```python
from build123d import *

# Parameters (mm, degrees)
SKETCH1_W                = 31
SKETCH1_H                = 14
BOSS_EXTRUDE1_DEPTH      = 6.6
SKETCH2_R                = 2.3
CUT_EXTRUDE1_DEPTH       = 1
ZAOBLIT7_R               = 3.3
ZAOBLIT12_R              = 3.3
ZAOBLIT13_R              = 3.3
ZAOBLIT14_R              = 3.3
ODEBRAT_START            = -1
SKICA1_R                 = 2.3
ODEBRAT_VYSUNUT_M1_DEPTH = 1
SKICA3_R                 = 2.3
ODEBRAT_VYSUNUT_M2_DEPTH = 3
ODEBRAT_VYSUNUT_M2_DRAFT = -15
SKICA4_R                 = 2.3
ODEBRAT_VYSUNUT_M3_DEPTH = 3
ODEBRAT_VYSUNUT_M3_DRAFT = -15
SKICA5_R                 = 2.3
ODEBRAT_VYSUNUT_M4_DEPTH = 3
ODEBRAT_VYSUNUT_M4_DRAFT = -15
SKICA6_R                 = 2.3
ODEBRAT_VYSUNUT_M5_DEPTH = 3
ODEBRAT_VYSUNUT_M5_DRAFT = -15


with BuildPart() as part:
    # Sketch1 → Boss-Extrude1 (new body)
    with BuildSketch(Plane.XY):
        with Locations((15.5, 7)):
            Rectangle(SKETCH1_W, SKETCH1_H)
    extrude(amount=BOSS_EXTRUDE1_DEPTH)

    # Sketch2 → Cut-Extrude1 (cut)
    with BuildSketch(Plane.ZY):
        with Locations((3.3, 10.7)):
            Circle(SKETCH2_R)
        with Locations((3.3, 3.3)):
            Circle(SKETCH2_R)
    extrude(amount=-CUT_EXTRUDE1_DEPTH, mode=Mode.SUBTRACT)

    # Zaoblit7
    zaoblit7_edges = [part.edges().sort_by_distance(p)[0] for p in [
        (15.5, 14, 0),
    ]]
    fillet(zaoblit7_edges, radius=ZAOBLIT7_R)

    # Zaoblit12
    zaoblit12_edges = [part.edges().sort_by_distance(p)[0] for p in [
        (15.5, 14, 6.6),
    ]]
    fillet(zaoblit12_edges, radius=ZAOBLIT12_R - 0.0001)  # a hair under: the kernel refuses the full size

    # Zaoblit13
    zaoblit13_edges = [part.edges().sort_by_distance(p)[0] for p in [
        (15.5, 0, 6.6),
    ]]
    fillet(zaoblit13_edges, radius=ZAOBLIT13_R)

    # Zaoblit14
    zaoblit14_edges = [part.edges().sort_by_distance(p)[0] for p in [
        (15.5, 0, 0),
    ]]
    fillet(zaoblit14_edges, radius=ZAOBLIT14_R - 0.0001)  # a hair under: the kernel refuses the full size

    # Skica1 → Odebrat vysunutím1 (cut)
    with BuildSketch(Plane(origin=(31, 0, 0), x_dir=(0, 0, -1), z_dir=(1, 0, 0)).offset(ODEBRAT_START)):
        with Locations(Location((-3.3, 10.7, 0), (0, 0, 180))):
            Circle(SKICA1_R)
        with Locations(Location((-3.3, 3.3, 0), (0, 0, 180))):
            Circle(SKICA1_R)
    extrude(amount=ODEBRAT_VYSUNUT_M1_DEPTH, mode=Mode.SUBTRACT)


with BuildPart() as odebrat_vysunut_m2_tool:
    # Skica3 → Odebrat vysunutím2 (with draft: the straight prism first)
    with BuildSketch(Plane.ZY.offset(-1)):
        with Locations((3.3, 10.7)):
            Circle(SKICA3_R)
    extrude(amount=-ODEBRAT_VYSUNUT_M2_DEPTH)
    # Odebrat vysunutím2: the draft: its side faces are tilted about the plane it starts from
    odebrat_vysunut_m2_sides = [odebrat_vysunut_m2_tool.faces().sort_by_distance(p)[0] for p in [
        (2.5, 10.7, 1),
    ]]
    draft(odebrat_vysunut_m2_sides, Plane.ZY.offset(-1), ODEBRAT_VYSUNUT_M2_DRAFT)


with BuildPart() as part_1:
    add(part.part)

    # Odebrat vysunutím2: cut by odebrat_vysunut_m2_tool
    add(odebrat_vysunut_m2_tool.part, mode=Mode.SUBTRACT)


with BuildPart() as odebrat_vysunut_m3_tool:
    # Skica4 → Odebrat vysunutím3 (with draft: the straight prism first)
    with BuildSketch(Plane.ZY.offset(-1)):
        with Locations((3.3, 3.3)):
            Circle(SKICA4_R)
    extrude(amount=-ODEBRAT_VYSUNUT_M3_DEPTH)
    # Odebrat vysunutím3: the draft: its side faces are tilted about the plane it starts from
    odebrat_vysunut_m3_sides = [odebrat_vysunut_m3_tool.faces().sort_by_distance(p)[0] for p in [
        (2.5, 3.3, 1),
    ]]
    draft(odebrat_vysunut_m3_sides, Plane.ZY.offset(-1), ODEBRAT_VYSUNUT_M3_DRAFT)


with BuildPart() as part_2:
    add(part_1.part)

    # Odebrat vysunutím3: cut by odebrat_vysunut_m3_tool
    add(odebrat_vysunut_m3_tool.part, mode=Mode.SUBTRACT)


with BuildPart() as odebrat_vysunut_m4_tool:
    # Skica5 → Odebrat vysunutím4 (with draft: the straight prism first)
    with BuildSketch(Plane(origin=(30, 0, 0), x_dir=(0, 0, -1), z_dir=(1, 0, 0))):
        with Locations(Location((-3.3, 10.7, 0), (0, 0, 180))):
            Circle(SKICA5_R)
    extrude(amount=-ODEBRAT_VYSUNUT_M4_DEPTH)
    # Odebrat vysunutím4: the draft: its side faces are tilted about the plane it starts from
    odebrat_vysunut_m4_sides = [odebrat_vysunut_m4_tool.faces().sort_by_distance(p)[0] for p in [
        (28.5, 10.7, 1),
    ]]
    draft(odebrat_vysunut_m4_sides, Plane(origin=(30, 0, 0), x_dir=(0, 0, -1), z_dir=(1, 0, 0)), ODEBRAT_VYSUNUT_M4_DRAFT)


with BuildPart() as part_3:
    add(part_2.part)

    # Odebrat vysunutím4: cut by odebrat_vysunut_m4_tool
    add(odebrat_vysunut_m4_tool.part, mode=Mode.SUBTRACT)


with BuildPart() as odebrat_vysunut_m5_tool:
    # Skica6 → Odebrat vysunutím5 (with draft: the straight prism first)
    with BuildSketch(Plane(origin=(30, 0, 0), x_dir=(0, 0, -1), z_dir=(1, 0, 0))):
        with Locations(Location((-3.3, 3.3, 0), (0, 0, 180))):
            Circle(SKICA6_R)
    extrude(amount=-ODEBRAT_VYSUNUT_M5_DEPTH)
    # Odebrat vysunutím5: the draft: its side faces are tilted about the plane it starts from
    odebrat_vysunut_m5_sides = [odebrat_vysunut_m5_tool.faces().sort_by_distance(p)[0] for p in [
        (28.5, 3.3, 1),
    ]]
    draft(odebrat_vysunut_m5_sides, Plane(origin=(30, 0, 0), x_dir=(0, 0, -1), z_dir=(1, 0, 0)), ODEBRAT_VYSUNUT_M5_DRAFT)


with BuildPart() as part_4:
    add(part_3.part)

    # Odebrat vysunutím5: cut by odebrat_vysunut_m5_tool
    add(odebrat_vysunut_m5_tool.part, mode=Mode.SUBTRACT)


solid = part_4.part
```
Here's how the part is built. I have some questions about the finished solid (model axes, mm). A direction names the side the tool comes from. Give positions to 0.01 mm unless a question says otherwise; leave off trailing zeros. Order: outer loops, then holes, each group sorted by start corner. A loop starts at its lowest first (then second) coordinate and runs counter-clockwise, first axis right, second up. Notation, with made-up numbers: (65.5, -12.75) -> (110.5, -12.75) arc R16 ccw to (110.5, 0.25) -> close; hole circle Ø1 at (18.25, 70.5). An arc over 180 degrees is marked (long way). Use CSV: the item, a comma, the result in double quotes. Start each with the question number.
Item 1: Thinking about a two-plate mould opening in Y: for faces 4 (the flat face through (4, 11, 3)), 5 (the cylindrical face through (15.717, 0.992, 5.659)), 6 (the flat face through (0, 7, 3)), which applies, pulls with the +Y half, pulls with the -Y half, needs draft (parallel to the pull), parting line crosses it, or undercut?
Item 2: I'm going to push flat-ended pins straight in: P1, Ø1, axis at x = 26.5, z = 0.5, coming from the +Y side; P2, Ø0.9, axis at y = 4, z = 3, coming from the +X side. Where does each tip first touch, or does it pass through?
Item 3: Suppose I cut it at B-B (z = 6.25). List the corners of the cut face in (x, y) for me, and give its area (3 significant figures).
Item 4: On a 3-axis mill with a long thin cutter (end or side, diameter ignored), from which of +Z, -Z, +X, -X, +Y, -Y can I reach the whole of each face in a straight line? I mean faces 1 (the cylindrical face through (0.493, 9.3, 1.475)), 2 (the cylindrical face through (15.717, 13.059, 5.608)), 3 (the flat face through (27, 3, 3)). Say none if no direction works.
Item 5: If I drill on probe 1 along X at (y, z) = (2.75, 4.25); probe 2 along Y at (x, z) = (16, 1.5); probe 3 along Y at (x, z) = (1, 6.25), over which ranges is the centre line in solid material (lowest first)? Write a range as [from, to].
Answer block:
1,face 4,"undercut"
1,face 5,"pulls with the -Y half"
1,face 6,"needs draft"
2,P1,"stops at y = 13.07"
2,P2,"stops at x = 27"
3,outline,"(0, 1.82) -> (31, 1.82) -> (31, 12.18) -> (0, 12.18) -> close"
3,area,"321 mm^2"
4,face 1,"-X"
4,face 2,"+Z, +X, -X, +Y"
4,face 3,"+X"
5,probe 1,"x = [4, 27]"
5,probe 2,"y = [0.53, 13.47]"
5,probe 3,"y = [1.82, 12.18]"
